from build123d import *

# Parameters (mm, degrees)
F0_W     = 1219.2
F0_H     = 787.4
F1_DEPTH = 12.7
F3_DEPTH = 12.701


with BuildPart() as f1:
    # F0 (on Front) → F1 (new body)
    with BuildSketch(Plane.XZ):
        Rectangle(F0_W, F0_H)
    extrude(amount=F1_DEPTH)

    # F2 (on face) → F3 (cut, through all)
    with BuildSketch(Plane.XZ.offset(12.7)):
        with BuildLine():
            ThreePointArc((-390.098016, 159.128398), (-447.001631, 178.590483), (-482.6, 130.118322))
            Line((-482.6, 130.118322), (-482.6, -215.9))
            ThreePointArc((-482.6, -215.9), (-460.281537, -269.781537), (-406.4, -292.1))
            Line((-406.4, -292.1), (-222.033056, -292.1))
            ThreePointArc((-222.033056, -292.1), (-154.4968, -251.188726), (-159.480079, -172.384886))
            Line((-159.480079, -172.384886), (-390.098016, 159.128398))
        make_face()
        with BuildLine():
            ThreePointArc((-230.670696, 292.1), (-275.694867, 264.825817), (-272.37268, 212.289924))
            Line((-272.37268, 212.289924), (-168.701984, 63.263298))
            ThreePointArc((-168.701984, 63.263298), (-111.798369, 43.801213), (-76.2, 92.273374))
            Line((-76.2, 92.273374), (-76.2, 241.3))
            ThreePointArc((-76.2, 241.3), (-91.078976, 277.221024), (-127, 292.1))
            Line((-127, 292.1), (-230.670696, 292.1))
        make_face()
        with BuildLine():
            ThreePointArc((76.2, 92.273374), (111.798369, 43.801213), (168.701984, 63.263298))
            Line((168.701984, 63.263298), (272.37268, 212.289924))
            ThreePointArc((272.37268, 212.289924), (275.694867, 264.825817), (230.670696, 292.1))
            Line((230.670696, 292.1), (127, 292.1))
            ThreePointArc((127, 292.1), (91.078976, 277.221024), (76.2, 241.3))
            Line((76.2, 241.3), (76.2, 92.273374))
        make_face()
        with BuildLine():
            ThreePointArc((482.6, 130.118322), (447.001631, 178.590483), (390.098016, 159.128398))
            Line((390.098016, 159.128398), (159.480079, -172.384886))
            ThreePointArc((159.480079, -172.384886), (154.4968, -251.188726), (222.033056, -292.1))
            Line((222.033056, -292.1), (406.4, -292.1))
            ThreePointArc((406.4, -292.1), (460.281537, -269.781537), (482.6, -215.9))
            Line((482.6, -215.9), (482.6, 130.118322))
        make_face()
    extrude(amount=-F3_DEPTH, mode=Mode.SUBTRACT)


solid = f1.part
Geometry: final body of the model. Coordinates: model frame, mm. A direction names the side the tool comes from. Give positions to 0.01 mm unless a question says otherwise; leave off trailing zeros. Loops run counter-clockwise (first coordinate to the right, second up) from the corner with the lowest first, then second, coordinate; pieces in that order, holes last. Notation, with made-up numbers: M 28,12.25 L 86,12.25 A30 cw 86,36.25 Z; hole C 88.25,22 d6. An arc over 180 degrees is marked long. Put each result on its own line as item: value. Start each with the question number.
1) Cut plane A-A (y = -5.25). Output: boundary loops of the cut face in (x, z).
2) Access query for faces 1 (the cylindrical face through (-90.686, -6.439, 276.824)), 2 (the flat face through (-9, 0, 6)). Directions: +Z, -Z, +X, -X, +Y, -Y. A direction counts if a zero-diameter tool reaches every point of the face in a straight line with its end or side. Return the directions, or none.
3) Cut plane C-C (z = -130). Output: boundary loops of the cut face in (x, y).
4) Pull-direction query (Z, two-part tool) for faces 3 (the flat face through (219.81, -6.44, 136.73)), 4 (the flat face through (-9, -12.7, 6)); classes: pulls with the +Z half, pulls with the -Z half, needs draft (parallel to the pull), parting line crosses it, or undercut.
5) Ray query, line 1 along X through (y, z) = (-2.5, -212.5); line 2 along X through (y, z) = (-8, -183.5); line 3 along Z through (x, y) = (-188.5, -2). Return the intervals inside material, ascending.
6) Cut plane B-B (x = 248). Output: boundary loops of the cut face in (y, z).
Verdict:
1. outline: M -609.6,-393.7 L 609.6,-393.7 L 609.6,393.7 L -609.6,393.7 Z; hole M -482.6,-215.9 A76.2 ccw -406.4,-292.1 L -222.03,-292.1 A76.2 ccw -159.48,-172.38 L -390.1,159.13 A50.8 ccw -482.6,130.12 Z; hole M -272.37,212.29 L -168.7,63.26 A50.8 ccw -76.2,92.27 L -76.2,241.3 A50.8 ccw -127,292.1 L -230.67,292.1 A50.8 ccw Z; hole M 76.2,92.27 A50.8 ccw 168.7,63.26 L 272.37,212.29 A50.8 ccw 230.67,292.1 L 127,292.1 A50.8 ccw 76.2,241.3 Z; hole M 159.48,-172.38 A76.2 ccw 222.03,-292.1 L 406.4,-292.1 A76.2 ccw 482.6,-215.9 L 482.6,130.12 A50.8 ccw 390.1,159.13 Z
2. face 1: +Y, -Y
2. face 2: +Z, -Z, +X, -X, +Y
3. outline: M -609.6,-12.7 L -482.6,-12.7 L -482.6,0 L -609.6,0 Z; M -188.97,-12.7 L 188.97,-12.7 L 188.97,0 L -188.97,0 Z; M 482.6,-12.7 L 609.6,-12.7 L 609.6,0 L 482.6,0 Z
4. face 3: undercut
4. face 4: needs draft
5. line 1: -609.6 to -482.6, -145.91 to 145.91, 482.6 to 609.6
5. line 2: -609.6 to -482.6, -153.06 to 153.06, 482.6 to 609.6
5. line 3: -393.7 to -284.32, -130.67 to 91.72, 292.1 to 393.7
6. outline: M -12.7,-393.7 L 0,-393.7 L 0,-292.1 L -12.7,-292.1 Z; M -12.7,-45.14 L 0,-45.14 L 0,177.25 L -12.7,177.25 Z; M -12.7,289.05 L 0,289.05 L 0,393.7 L -12.7,393.7 Z
